```python
from build123d import *

# Parameters (mm, degrees)
SKETCH1_W                           = 38.1
SKETCH1_H                           = 63.5
MAIN_BODY_DEPTH                     = 3.175
SKETCH2_W                           = 3.2258
SKETCH2_H                           = 6.35
TABS_DEPTH                          = 3.175
SKETCH5_R                           = 1.7145
MOTOR_CUT_DEPTH                     = 4.175
SKETCH6_R                           = 3.2385
CUT_FOR_AXLE_DEPTH                  = 4.175
ROUND_OFF_BACK_CORNER_DEPTH         = 4.175
SKETCH9_W                           = 3.2258
SKETCH9_H                           = 6.35
CUT_FOR_TABS_DEPTH                  = 4.175
SKETCH10_R                          = 3.048
CUT_FOR_SCREW_ACCESS_DEPTH          = 4.175
SKETCH11_R                          = 1.5875
CUT_FOR_BRACKET_SCREW_DEPTH         = 4.175
SKETCH12_R                          = 1.5875
CUT_FOR_BASIC_TILT_LOCK_SCREW_DEPTH = 4.175


with BuildPart() as part:
    # Sketch1 → main body (new body)
    with BuildSketch(Plane(origin=(0, 0, 0), x_dir=(0, 0, -1), z_dir=(1, 0, 0))):
        Rectangle(SKETCH1_W, SKETCH1_H)
    extrude(amount=MAIN_BODY_DEPTH)

    # Sketch2 → tabs (add)
    with BuildSketch(Plane(origin=(3.175, 0, 0), x_dir=(0, 0, -1), z_dir=(1, 0, 0))):
        with Locations((-20.6629, 22.225)):
            Rectangle(SKETCH2_W, SKETCH2_H)
        with Locations((-20.6629, -3.175)):
            Rectangle(SKETCH2_W, SKETCH2_H)
    extrude(amount=-TABS_DEPTH)

    # Sketch5 → motor cut (cut, through all)
    with BuildSketch(Plane(origin=(3.175, 0, 0), x_dir=(0, 0, -1), z_dir=(1, 0, 0))):
        with Locations((1.905, -20.32)):
            Circle(SKETCH5_R)
    extrude(amount=-MOTOR_CUT_DEPTH, mode=Mode.SUBTRACT)

    # Sketch6 → cut for axle (cut, through all)
    with BuildSketch(Plane(origin=(3.175, 0, 0), x_dir=(0, 0, -1), z_dir=(1, 0, 0))):
        with Locations((-1.27, 23.495)):
            Circle(SKETCH6_R)
    extrude(amount=-CUT_FOR_AXLE_DEPTH, mode=Mode.SUBTRACT)

    # Sketch7 → round off back corner (cut, through all)
    with BuildSketch(Plane(origin=(3.175, 0, 0), x_dir=(0, 0, -1), z_dir=(1, 0, 0))):
        with BuildLine():
            Line((19.05, -31.75), (19.05, -6.35))
            ThreePointArc((19.05, -6.35), (15.925359096, -20.215661593), (7.62, -31.75))
            Line((7.62, -31.75), (19.05, -31.75))
        make_face()
    extrude(amount=-ROUND_OFF_BACK_CORNER_DEPTH, mode=Mode.SUBTRACT)

    # Sketch9 → cut for tabs (cut, through all)
    with BuildSketch(Plane(origin=(3.175, 0, 0), x_dir=(0, 0, -1), z_dir=(1, 0, 0))):
        with Locations((14.2113, 22.225)):
            Rectangle(SKETCH9_W, SKETCH9_H)
        with Locations((14.2113, 6.985)):
            Rectangle(SKETCH9_W, SKETCH9_H)
    extrude(amount=-CUT_FOR_TABS_DEPTH, mode=Mode.SUBTRACT)

    # Sketch10 → cut for screw access (cut, through all)
    with BuildSketch(Plane.ZY):
        with Locations((6.35, -1.27)):
            Circle(SKETCH10_R)
    extrude(amount=-CUT_FOR_SCREW_ACCESS_DEPTH, mode=Mode.SUBTRACT)

    # Sketch11 → cut for bracket screw (cut, through all)
    with BuildSketch(Plane.ZY):
        with Locations((12.7, 15.24)):
            Circle(SKETCH11_R)
    extrude(amount=-CUT_FOR_BRACKET_SCREW_DEPTH, mode=Mode.SUBTRACT)

    # Sketch12 → cut for basic tilt lock screw (cut, through all)
    with BuildSketch(Plane.ZY):
        with Locations((-9.398, 18.0975)):
            Circle(SKETCH12_R)
    extrude(amount=-CUT_FOR_BASIC_TILT_LOCK_SCREW_DEPTH, mode=Mode.SUBTRACT)


solid = part.part
```
Geometry: final body of the model. Coordinates: model frame, mm. A direction names the side the tool comes from. Coordinates: 2 decimals unless noted, no trailing zeros. Order: outer loops, then holes, each group sorted by start corner. A loop starts at its lowest first (then second) coordinate and runs counter-clockwise, first axis right, second up. Notation, with made-up numbers: M 64.5,23.5 L 91.5,23.5 A21 ccw 91.5,46.5 Z; hole C 12.25,-34 d9. An arc over 180 degrees is marked long. Answer in a Markdown table with one row per item. Add a question column.
Q1. Mould query, pull axis Y, two halves, no side actions, for faces 1 (the flat face through (0, 0, 2)), 2 (the cylindrical face through (1.565, 19.671, -9.605)), 3 (the cylindrical face through (1.61, -20.03, -16.01)), 4 (the flat face through (2, 7, -15.824)). Classes: released by +Y, released by -Y, zero draft, split by the parting line, or undercut.
Q2. Reachability of faces 5 (the flat face through (2, -31.75, 6)), 6 (the flat face through (2, 22, -15.824)), 7 (the flat face through (2, -6.35, 21)), 8 (the flat face through (2, 25.4, 21)) from +Z, -Z, +X, -X, +Y, -Y: full face, straight path, thin tool, end or side. Return the list, or none.
Q3. Line query: L1, parallel to Y at x = 0.9, z = 6.35; L2, parallel to Z at x = 1.95, y = 22; L3, parallel to Z at x = 1.3, y = 5. Output: solid intervals per line, ascending.
Q4. Section query D-D on y = -14. Return the cut outline in (x, z) (3 decimals), and give its area (3 significant figures).
Q5. Section query C-C on x = 1.7. Count the separate pieces of the cut face and the enclosed holes in it, and give its area (3 significant figures).
Q6. Contact query for flat-ended pins moving along their axis: P1, Ø1.6, axis at x = 1, z = -14.5, coming from the -Y side; P2, Ø1, axis at x = 1, y = 28, coming from the +Z side. Output: stop coordinate, or through.
Completed:
| question | item | result |
|---|---|---|
| 1 | face 1 | zero draft |
| 1 | face 2 | undercut |
| 1 | face 3 | released by -Y |
| 1 | face 4 | undercut |
| 2 | face 5 | +Z, -Z, +X, -X, -Y |
| 2 | face 6 | +X, -X |
| 2 | face 7 | +Z, +X, -X, -Y |
| 2 | face 8 | +Z, +X, -X, +Y |
| 3 | L1 | y = -31.75 to -4.32, 1.78 to 31.75 |
| 3 | L2 | z = -19.05 to -15.82, -12.6 to -1.6, 4.14 to 22.28 |
| 3 | L3 | z = -19.05 to -15.82, -12.6 to 19.05 |
| 4 | outline | M 0,-18.057 L 3.175,-18.057 L 3.175,19.05 L 0,19.05 Z |
| 4 | area | 118 mm2 |
| 5 | separate pieces | 1 |
| 5 | enclosed holes | 7 |
| 5 | area | 2,240 mm2 |
| 6 | P1 | stops at y = -24.39 |
| 6 | P2 | stops at z = 19.05 |
